from build123d import *

# Parameters (mm, degrees)
CROQUIS1_R              = 1.55
CROQUIS1_R_2            = 4
SALIENTE_EXTRUIR1_DEPTH = 120
CORTAR_EXTRUIR1_DEPTH   = 117


with BuildPart() as part:
    # Croquis1 → Saliente-Extruir1 (new body)
    with BuildSketch(Plane(origin=(0, 0, 0), x_dir=(1, 0, 0), z_dir=(0, 1, 0))):
        Polygon((17, -7.04163056), (17, 7.04163056), (7.04163056, 17), (-7.04163056, 17), (-17, 7.04163056), (-17, -7.04163056), (-7.04163056, -17), (7.04163056, -17), align=None)
        with Locations(Location((0, 11, 0), (0, 0, 270))):
            Circle(CROQUIS1_R, mode=Mode.SUBTRACT)
        with Locations(Location((0, 0, 0), (0, 0, 270))):
            Circle(CROQUIS1_R_2, mode=Mode.SUBTRACT)
        with Locations(Location((7.778174593, 7.778174593, 0), (0, 0, 270))):
            Circle(CROQUIS1_R, mode=Mode.SUBTRACT)
        with Locations(Location((11, 0, 0), (0, 0, 270))):
            Circle(CROQUIS1_R, mode=Mode.SUBTRACT)
        with Locations(Location((7.778174593, -7.778174593, 0), (0, 0, 270))):
            Circle(CROQUIS1_R, mode=Mode.SUBTRACT)
        with Locations(Location((0, -11, 0), (0, 0, 270))):
            Circle(CROQUIS1_R, mode=Mode.SUBTRACT)
        with Locations(Location((-7.778174593, -7.778174593, 0), (0, 0, 270))):
            Circle(CROQUIS1_R, mode=Mode.SUBTRACT)
        with Locations(Location((-11, 0, 0), (0, 0, 270))):
            Circle(CROQUIS1_R, mode=Mode.SUBTRACT)
        with Locations(Location((-7.778174593, 7.778174593, 0), (0, 0, 270))):
            Circle(CROQUIS1_R, mode=Mode.SUBTRACT)
    extrude(amount=SALIENTE_EXTRUIR1_DEPTH)

    # Croquis2 → Cortar-Extruir1 (cut)
    with BuildSketch(Plane(origin=(0, 120, 0), x_dir=(1, 0, 0), z_dir=(0, 1, 0))):
        Polygon((6.213203436, 15), (-6.213203436, 15), (-15, 6.213203436), (-15, -6.213203436), (-6.213203436, -15), (6.213203436, -15), (15, -6.213203436), (15, 6.213203436), align=None)
    extrude(amount=-CORTAR_EXTRUIR1_DEPTH, mode=Mode.SUBTRACT)


solid = part.part
Model file for the job. Use its own axes, mm. A direction names the side the tool comes from. Give positions to 0.01 mm unless a question says otherwise; leave off trailing zeros. Order: outer loops, then holes, each group sorted by start corner. A loop starts at its lowest first (then second) coordinate and runs counter-clockwise, first axis right, second up. Notation, with made-up numbers: (-1.75, -29) - (25.25, -29) arc R25 ccw to (25.25, 7) - close; hole circle Ø7 at (37, 56). An arc over 180 degrees is marked (long way). Return JSON: item names as keys, results as strings.
1) Cut at B-B, the plane y = 90.5. Give the cut face in (x, z).
Geometry says:
{"outline": "(-17, -7.04) - (-7.04, -17) - (7.04, -17) - (17, -7.04) - (17, 7.04) - (7.04, 17) - (-7.04, 17) - (-17, 7.04) - close; hole (-15, -6.21) - (-6.21, -15) - (6.21, -15) - (15, -6.21) - (15, 6.21) - (6.21, 15) - (-6.21, 15) - (-15, 6.21) - close"}
2) Flat gauge pins, fed straight in: P1, Ø2.5, axis at x = 0, z = -11, coming from the -Y side; P2, Ø4, axis at x = 7.78, z = 7.78, coming from the -Y side; P3, Ø15, axis at x = 2.5, z = -3.5, coming from the +Y side. Where does each tip first touch, or does it go through?
Geometry says:
{"P1": "through", "P2": "y = 0", "P3": "y = 3"}
3) Cut at C-C, the plane z = 10.5. Give the cut face in (x, y), plus the area to 3 significant figures.
Geometry says:
{"outline": "(-13.54, 0) - (-1.47, 0) - (-1.47, 3) - (-10.71, 3) - (-10.71, 120) - (-13.54, 120) - close; (1.47, 0) - (13.54, 0) - (13.54, 120) - (10.71, 120) - (10.71, 3) - (1.47, 3) - close", "area": "734 mm²"}
4) Pull direction X, two halves, no side cores. Call faces 1 (the flat face through (-10.668, 62.319, 10.545)), 2 (the flat face through (17, 59, 0)), 3 (the flat face through (0, 59, 17)): pulls with the +X half, pulls with the -X half, needs draft (parallel to the pull), parting line crosses it, or undercut.
Geometry says:
{"face 1": "undercut", "face 2": "pulls with the +X half", "face 3": "needs draft"}
5) Probe line 1 (Z direction, x = 0, y = 2.3); line 2 (X direction, y = 53.5, z = -3.5). List the from-to ranges inside material, lowest first. Write a range as from..to.
Geometry says:
{"line 1": "-17..-12.55, -9.45..-4, 4..9.45, 12.55..17", "line 2": "-17..-15, 15..17"}
6) 3-axis set-ups, long thin cutter, end or side, ignore diameter. For faces 4 (the cylindrical face through (-6.73, 1.48, -8.92)), 5 (the flat face through (-15, 62, 0)): which of +Z, -Z, +X, -X, +Y, -Y reach the whole face in a straight line?
Geometry says:
{"face 4": "+Y, -Y", "face 5": "+Y"}
7) Cut at A-A, the plane x = 0. Give the cut face in (y, z), plus the area to 3 significant figures.
Geometry says:
{"outline": "(0, -17) - (120, -17) - (120, -15) - (3, -15) - (3, -12.55) - (0, -12.55) - close; (0, -9.45) - (3, -9.45) - (3, -4) - (0, -4) - close; (0, 4) - (3, 4) - (3, 9.45) - (0, 9.45) - close; (0, 12.55) - (3, 12.55) - (3, 15) - (120, 15) - (120, 17) - (0, 17) - close", "area": "527 mm²"}
8) Cut at D-D, the plane x = 11. Give the cut face in (y, z), plus the area to 3 significant figures.
Geometry says:
{"outline": "(0, -13.04) - (120, -13.04) - (120, -10.21) - (3, -10.21) - (3, -1.55) - (0, -1.55) - close; (0, 1.55) - (3, 1.55) - (3, 10.21) - (120, 10.21) - (120, 13.04) - (0, 13.04) - close", "area": "731 mm²"}
